Work out the finished part from the listing and answer in its coordinate system (mm). A direction names the side the tool comes from. Round coordinates to 2 decimals unless told otherwise and drop trailing zeros. Write each loop counter-clockwise with the first axis right and the second up, starting at its lowest first coordinate (ties: lowest second). Pieces come first, ordered by that corner, then holes. Notation, with made-up numbers: (-2.5, 76.25) -> (21.5, 76.25) arc R34 cw to (21.5, 115.25) -> close; hole circle Ø9 at (21.25, 33). An arc over 180 degrees is marked (long way). One line per item, written item: value.
```python
from build123d import *

# Parameters (mm, degrees)
F1_DEPTH = 19.05
F2_DEPTH = 19.05
F3_R     = 9.525
F4_DEPTH = 25
F5_W     = 19.05
F5_H     = 38.1
F6_DEPTH = 285.75
F9_DEPTH = 38.1


# Not quite as in the source:
# - a feature names something its author has since deleted; it is built from what else it names


with BuildPart() as f1:
    # F0 (on Front) → F1 (new body)
    with BuildSketch(Plane.XZ):
        Polygon((435.2484990698, 38.1), (-435.2484990698, 38.1), (-456.4151657365, 0), (456.4151657365, 0), align=None)
    extrude(amount=F1_DEPTH)

    # F0 (on Front) → F2 (join)
    with BuildSketch(Plane.XZ):
        Polygon((500, 0), (478.8333333333, 38.1), (435.2484990698, 38.1), (456.4151657365, 0), align=None)
        Polygon((478.8333333333, 38.1), (21.7924171318, 860.7736491628), (0, 821.5472983257), (435.2484990698, 38.1), align=None)
        Polygon((21.7924171318, 860.7736491628), (0, 900), (-21.7924171318, 860.7736491628), (0, 821.5472983257), align=None)
        Polygon((0, 821.5472983257), (-21.7924171318, 860.7736491628), (-478.8333333333, 38.1), (-435.2484990698, 38.1), align=None)
        Polygon((-435.2484990698, 38.1), (-478.8333333333, 38.1), (-500, 0), (-456.4151657365, 0), align=None)
    extrude(amount=F2_DEPTH)

    # F3 (on face) → F4 (cut)
    with BuildSketch(Plane.XZ.offset(19.05)):
        with Locations((0, 860.7736491628)):
            Circle(F3_R)
    extrude(amount=-F4_DEPTH, mode=Mode.SUBTRACT)

    # F5 (on face) → F6 (join)
    with BuildSketch(Plane.XZ.offset(19.05)):
        with Locations((-425.7234990698, 19.05)):
            Rectangle(F5_W, F5_H)
        with Locations((425.7234990698, 19.05)):
            Rectangle(F5_W, F5_H)
    extrude(amount=F6_DEPTH)

    # F7: F1 across face


with BuildPart() as f1_1:
    add(f1.part)
    add(f1.part.mirror(Plane(origin=(425.7234990698, -304.8, 19.05), x_dir=(1, 0, 0), z_dir=(0, -1, 0))))

    # F8 (on Top) → F9 (join, through all)
    with BuildSketch(Plane.XY):
        Polygon((416.1984990698, -590.55), (-416.1984990698, -19.05), (-416.1984990698, -42.1577389905), (382.5417841626, -590.55), align=None)
    extrude(amount=F9_DEPTH)


solid = f1_1.part
```
(1) Find section A-A on x = -335. Give the vertices of the cut face in (y, z), plus the area to 3 significant figures.
Reported:
outline: (-609.6, 0) -> (-590.55, 0) -> (-590.55, 38.1) -> (-609.6, 38.1) -> close; (-609.6, 218.55) -> (-590.55, 218.55) -> (-590.55, 297) -> (-609.6, 297) -> close; (-97.91, 0) -> (-74.8, 0) -> (-74.8, 38.1) -> (-97.91, 38.1) -> close; (-19.05, 0) -> (0, 0) -> (0, 38.1) -> (-19.05, 38.1) -> close; (-19.05, 218.55) -> (0, 218.55) -> (0, 297) -> (-19.05, 297) -> close
area: 5,320 mm2
(2) Find section C-C on z = 657.5. Give the vertices of the cut face in (x, y), plus the area to 3 significant figures.
Reported:
outline: (-134.72, -609.6) -> (-91.14, -609.6) -> (-91.14, -590.55) -> (-134.72, -590.55) -> close; (-134.72, -19.05) -> (-91.14, -19.05) -> (-91.14, 0) -> (-134.72, 0) -> close; (91.14, -609.6) -> (134.72, -609.6) -> (134.72, -590.55) -> (91.14, -590.55) -> close; (91.14, -19.05) -> (134.72, -19.05) -> (134.72, 0) -> (91.14, 0) -> close
area: 3,320 mm2
(3) Flat-ended cylindrical pins translate along their axes: pin 1 Ø11.5 at (y, z) = (-180.5, 27.5) entering from -X; pin 2 Ø19 at (y, z) = (-375, 12.5) entering from +X; pin 3 Ø15 at (x, z) = (0, 860.77) entering from +Y. Find the tip coordinate at first contact, or state that the pin passes through.
Reported:
pin 1: stops at x = -435.25
pin 2: stops at x = 435.25
pin 3: passes through
(4) Consider probe 1 along Z at (x, y) = (0, -602); probe 2 along Y at (x, z) = (-206, 469). Determine where each line is inside the solid, lowest interval first.
Reported:
probe 1: z = 0 to 38.1, 821.55 to 851.25, 870.3 to 900
probe 2: y = -609.6 to -590.55, -19.05 to 0
(5) For a pull along Z with two mould halves and no side action, classify faces 6 (the face through (214.578, -600.208, 435.308)), 7 (the face through (-22.42, -312.515, 18.783)), 8 (the face through (-246.5, -600.2, 456.3)) as pulls with the +Z half, pulls with the -Z half, needs draft (parallel to the pull), parting line crosses it, or undercut.
Reported:
face 6: undercut
face 7: needs draft
face 8: pulls with the +Z half
(6) A tool of negligible diameter and unlimited length cuts with its end or side. For faces 1 (the face through (-435.248, -309, 19)), 2 (the face through (-2, -326, 0)), 3 (the face through (435.248, -309, 19)), 4 (the face through (-22, -590.55, 19)), 5 (the face through (-220.67, -600.21, 424.34)), from which of +Z, -Z, +X, -X, +Y, -Y can it reach the whole face along a straight path? Write none if from no direction.
Reported:
face 1: +Z, -Z, -X
face 2: -Z, +X, -X, +Y, -Y
face 3: +Z, -Z, +X
face 4: +Z, -Z
face 5: +Y, -Y
(7) Find section B-B on y = -261. Give the vertices of the cut face in (x, z).
Reported:
outline: (-435.25, 0) -> (-416.2, 0) -> (-416.2, 38.1) -> (-435.25, 38.1) -> close; (-97.45, 0) -> (-63.8, 0) -> (-63.8, 38.1) -> (-97.45, 38.1) -> close; (416.2, 0) -> (435.25, 0) -> (435.25, 38.1) -> (416.2, 38.1) -> close
